Input: part model. Units: mm. Frame: model coordinates. A direction names the side the tool comes from. Coordinates: 2 decimals unless noted, no trailing zeros. Loops run counter-clockwise (first coordinate to the right, second up) from the corner with the lowest first, then second, coordinate; pieces in that order, holes last. Notation, with made-up numbers: (-39, -17) - (-4, -17) arc R21 cw to (-4, 17) - close; hole circle Ø9 at (-25, 78.5). An arc over 180 degrees is marked (long way). Use a Markdown table: item, result. Add a question column.
1. Access query for faces 1 (the face through (-2.074, 20.07, -10.715)), 2 (the face through (2.325, 20.07, -9.285)), 3 (the face through (0, 20, -9)), 4 (the face through (0, 20, -11)), 5 (the face through (2.34, 20.07, -10.7)). Directions: +Z, -Z, +X, -X, +Y, -Y. A direction counts if a zero-diameter tool reaches every point of the face in a straight line with its end or side. Return the directions, or none.
2. Section query A-A on x = 0. Return the cut outline in (y, z), then the cut area to 3 significant figures.
3. Ray query, L1, parallel to Y at x = 14, z = -1.5; L2, parallel to X at y = 6.25, z = -0.5; L3, parallel to X at y = 3.75, z = -9.5. Return the intervals inside material, ascending. Write a range as [from, to].
4. Section query C-C on z = 0. Return the cut outline in (x, y).
5. Contact query for flat-ended pins moving along their axis: P1, Ø12, axis at x = 8, z = -6.5, coming from the -Y side; P2, Ø12, axis at x = 2, z = -2, coming from the +Y side; P3, Ø2, axis at x = -13, y = 6, coming from the -Z side; P4, Ø12, axis at y = 16, z = -9, coming from the -X side. Output: stop coordinate, or through.
6. Section query D-D on y = 1.5. Return the cut outline in (x, z).
```python
from build123d import *

# Parameters (mm, degrees)
SKETCH1_R           = 20
BOSS_EXTRUDE1_DEPTH = 15
SKETCH2_W           = 5
SKETCH2_H           = 2
BOSS_EXTRUDE2_DEPTH = 10
FILLET1_R           = 1


with BuildPart() as part:
    # Sketch1 → Boss-Extrude1 (new body)
    with BuildSketch(Plane(origin=(0, 0, 0), x_dir=(1, 0, 0), z_dir=(0, 1, 0))):
        with Locations(Location((0, 0, 0), (0, 0, 270))):
            Circle(SKETCH1_R)
    extrude(amount=BOSS_EXTRUDE1_DEPTH)

    # Sketch2 → Boss-Extrude2 (add)
    with BuildSketch(Plane(origin=(0, 15, 0), x_dir=(1, 0, 0), z_dir=(0, 1, 0))):
        with Locations((0.125263177, 10)):
            Rectangle(SKETCH2_W, SKETCH2_H)
    extrude(amount=BOSS_EXTRUDE2_DEPTH)

    # Fillet1
    fillet1_edges = [part.edges().sort_by_distance(p)[0] for p in [
        (-2.374736823, 20, -11),
        (2.625263177, 20, -11),
        (-2.374736823, 20, -9),
        (2.625263177, 20, -9),
    ]]
    fillet(fillet1_edges, radius=FILLET1_R - 0.0001)  # a hair under: the kernel refuses the full size


solid = part.part
```
Resolved:
| question | item | result |
|---|---|---|
| 1 | face 1 | -Z, -X, +Y |
| 1 | face 2 | +Z, +X, +Y |
| 1 | face 3 | +Z, +X, -X, +Y |
| 1 | face 4 | -Z, +X, -X, +Y |
| 1 | face 5 | -Z, +X, +Y |
| 2 | outline | (0, -20) - (15, -20) - (15, -11) - (25, -11) - (25, -9) - (15, -9) - (15, 20) - (0, 20) - close |
| 2 | area | 620 mm² |
| 3 | L1 | [0, 15] |
| 3 | L2 | [-19.99, 19.99] |
| 3 | L3 | [-17.6, 17.6] |
| 4 | outline | (-20, 0) - (20, 0) - (20, 15) - (-20, 15) - close |
| 5 | P1 | y = 0 |
| 5 | P2 | y = 15 |
| 5 | P3 | z = -16 |
| 5 | P4 | x = -19.76 |
| 6 | outline | circle Ø40 at (0, 0) |
